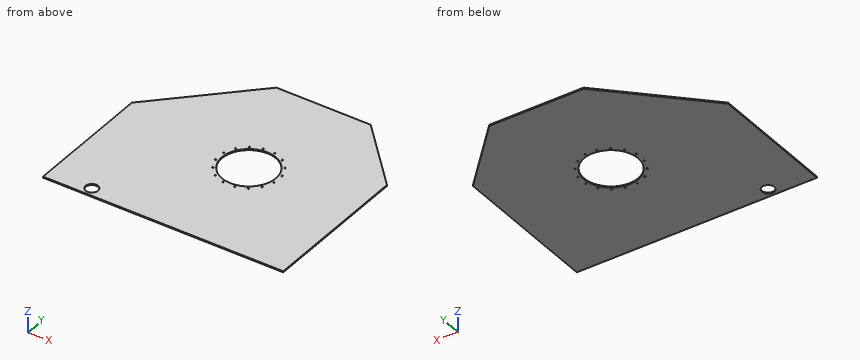
Autodesk Inventor part; units mm, degrees
ref_plane "YZ Plane" through (0, 0, 0) normal (1, 0, 0) x (0, 1, 0)
ref_plane "XZ Plane" through (0, 0, 0) normal (0, 1, 0) x (-1, 0, 0)
ref_plane "XY Plane" through (0, 0, 0) normal (0, 0, 1) x (1, 0, 0)
sketch "Sketch1" plane through (0, 0, 0) normal (0, 0, 1) x (1, 0, 0)
  line L0 (0, 0) -> (0, 1910) construction
  line L1 (424.5155, 1910) -> (-415.4845, 1910)
  line L2 (-415.4845, 1910) -> (-1180, 1150)
  line L3 (-1180, 0) -> (-1180, 1150)
  line L4 (960, 0) -> (960, 1342.8524)
  line L5 (424.5155, 1910) -> (960, 1342.8524)
  circle A0 centre (0, 950) radius 265 construction
  line L6 (960, 0) -> (-1180, 0)
  circle A1 centre (-1701.6377, -269.2167) radius 188.5 construction
  circle A2 centre (-800, 80) radius 55.5
  circle A3 centre (0, 950) radius 240
  line L7 (0, 1215) -> (0, 1190) construction
  circle A4 centre (51.6989, 1209.9081) radius 5.5
  line L8 (0, 950) -> (51.6989, 1209.9081) construction
  circle A5 centre (-51.6989, 1209.9081) radius 5.5
  circle A6 centre (-147.2261, 1170.3394) radius 5.5
  circle A7 centre (-220.3394, 1097.2261) radius 5.5
  circle A8 centre (-259.9081, 1001.6989) radius 5.5
  circle A9 centre (-259.9081, 898.3011) radius 5.5
  circle A10 centre (-220.3394, 802.7739) radius 5.5
  circle A11 centre (-147.2261, 729.6606) radius 5.5
  circle A12 centre (-51.6989, 690.0919) radius 5.5
  circle A13 centre (51.6989, 690.0919) radius 5.5
  circle A14 centre (147.2261, 729.6606) radius 5.5
  circle A15 centre (220.3394, 802.7739) radius 5.5
  circle A16 centre (259.9081, 898.3011) radius 5.5
  circle A17 centre (259.9081, 1001.6989) radius 5.5
  circle A18 centre (220.3394, 1097.2261) radius 5.5
  circle A19 centre (147.2261, 1170.3394) radius 5.5
  dimension "d72" = 480
  dimension "d1" = 840
  dimension "d3" = 1150
  dimension "d12" = 1180
  dimension "d13" = 950
  dimension "d14" = 111
  dimension "d15" = 1910
  dimension "d17" = -521.6377
  dimension "d18" = 377
  dimension "d19" = -269.2167
  dimension "d34" = 380
  dimension "d35" = 80
  dimension "d37" = 2140
  dimension "d52" = 530
  dimension "d69" = 780
  dimension "d71" = 1078
  dimension "d74" = 11
  dimension "d79" = 11.25
  dimension "d82" = 360
extrude "Extrusion1" add sketch "Sketch1" along normal blind 10
fillet "Fillet1" [suppressed]
sketch "Sketch4" plane through (0, 0, 0) normal (0, 0, 1) x (1, 0, 0)
  circle A0 centre (-51.6989, 1209.9081) radius 6.5
  circle A1 centre (0, 950) radius 240
  line L0 (0, 950) -> (0, 1196.7062) construction
  line L1 (-51.6989, 1209.9081) -> (0, 950) construction
  point P0 (0, 0)
  point P1 (240, 950)
  point P2 (-5, 1149.9375)
  point P3 (-2.5, 1189.987)
  point P4 (-168.8194, 970)
  point P5 (-2.5, 710.013)
  dimension "d59" = 265
  dimension "d60" = 13
  dimension "d61" = 11.25
extrude "Extrusion4" [suppressed]
pattern_circular "Circular Pattern3" [suppressed]
properties part number "Wall right v2.0"
The listing builds one solid part. Answer for the finished solid, in the listing's coordinates (mm). Coordinates: 2 decimals unless noted, no trailing zeros. Order: outer loops, then holes, each group sorted by start corner. A loop starts at its lowest first (then second) coordinate and runs counter-clockwise, first axis right, second up.
Q1. Consider line 1 (Y direction, x = 151, z = 5.75); line 2 (Y direction, x = 210, z = 1.75); line 3 (X direction, y = 749.5, z = 0.75). Determine where each line is inside the solid, lowest interval first.
Q2. A cutting plane is placed at C-C, the plane z = 8.25. State how many separate pieces and enclosed holes the cut face has, and give its area (3 significant figures).
Q3. A cutting plane is placed at B-B, the plane x = 0. Write down the section's boundary in (y, z), and give its area (3 significant figures).
Q4. A cutting plane is placed at D-D, the plane y = 1535.5. Write down the section's boundary in (x, z), and give its area (3 significant figures).
Q5. A cutting plane is placed at A-A, the plane y = 80. Write down the section's boundary in (x, z), and give its area (3 significant figures).
Answers follow:
1. line 1: y = 0 to 725.66, 733.66 to 763.46, 1136.54 to 1166.34, 1174.34 to 1910
1. line 2: y = 0 to 833.81, 1066.19 to 1910
1. line 3: x = -1180 to -131.91, 131.91 to 960
2. separate pieces: 1
2. enclosed holes: 18
2. area: 3,450,000 mm2
3. outline: (0, 0) - (710, 0) - (710, 10) - (0, 10) - close; (1190, 0) - (1910, 0) - (1910, 10) - (1190, 10) - close
3. area: 14,300 mm2
4. outline: (-792.21, 0) - (778.11, 0) - (778.11, 10) - (-792.21, 10) - close
4. area: 15,700 mm2
5. outline: (-1180, 0) - (-855.5, 0) - (-855.5, 10) - (-1180, 10) - close; (-744.5, 0) - (960, 0) - (960, 10) - (-744.5, 10) - close
5. area: 20,300 mm2
